The figure shows three views and two pictorial views of one solid part (mm, origin at its lowest corner). Answer the questions. Give positions to 0.01 mm unless a question says otherwise; leave off trailing zeros. Order: outer loops, then holes, each group sorted by start corner. A loop starts at its lowest first (then second) coordinate and runs counter-clockwise, first axis right, second up. Notation, with made-up numbers: (53.5, 76.25) - (97.5, 76.25) arc R23 ccw to (97.5, 86.25) - close; hole circle Ø5 at (61, 4.5). An arc over 180 degrees is marked (long way). Use a Markdown table: item, result. Add a question column.
1. A cutting plane is placed at B-B on z = 3.65. Determine the outline of the cut face in (x, y), and give its area (3 significant figures).
2. A cutting plane is placed at C-C on x = 38. Determine the outline of the cut face in (y, z).
3. A cutting plane is placed at D-D on x = 15.5. Determine the outline of the cut face in (y, z).
4. A cutting plane is placed at A-A on y = 10.5. Determine the outline of the cut face in (x, z), and give its area (3 significant figures).
5. Consider L1, parallel to X at y = 12.75, z = 2.55; L2, parallel to X at y = 10.5, z = 3.1; L3, parallel to Y at x = 38, z = 1.1. Determine where each line is inside the solid, lowest interval first.
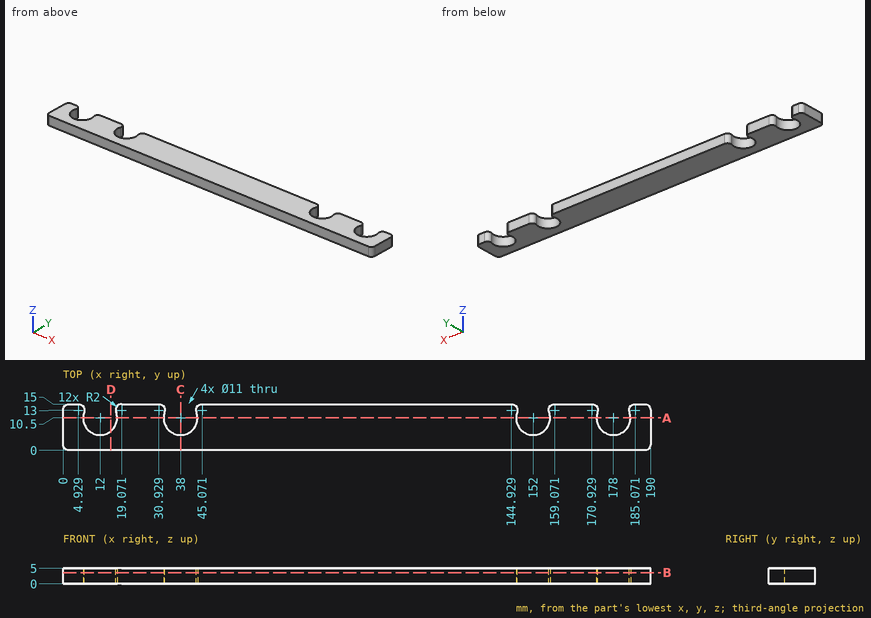
Output values:
| question | item | result |
|---|---|---|
| 1 | outline | (0, 2) arc R2 ccw to (2, 0) - (188, 0) arc R2 ccw to (190, 2) - (190, 13) arc R2 ccw to (188, 15) - (185.07, 15) arc R2 ccw to (183.19, 12.33) arc R5.5 cw (long way) to (172.81, 12.33) arc R2 ccw to (170.93, 15) - (159.07, 15) arc R2 ccw to (157.19, 12.33) arc R5.5 cw (long way) to (146.81, 12.33) arc R2 ccw to (144.93, 15) - (45.07, 15) arc R2 ccw to (43.19, 12.33) arc R5.5 cw (long way) to (32.81, 12.33) arc R2 ccw to (30.93, 15) - (19.07, 15) arc R2 ccw to (17.19, 12.33) arc R5.5 cw (long way) to (6.81, 12.33) arc R2 ccw to (4.93, 15) - (2, 15) arc R2 ccw to (0, 13) - close |
| 1 | area | 2,460 mm² |
| 2 | outline | (0, 0) - (5, 0) - (5, 5) - (0, 5) - close |
| 3 | outline | (0, 0) - (6.26, 0) - (6.26, 5) - (0, 5) - close |
| 4 | outline | (0, 0) - (6.5, 0) - (6.5, 5) - (0, 5) - close; (17.5, 0) - (32.5, 0) - (32.5, 5) - (17.5, 5) - close; (43.5, 0) - (146.5, 0) - (146.5, 5) - (43.5, 5) - close; (157.5, 0) - (172.5, 0) - (172.5, 5) - (157.5, 5) - close; (183.5, 0) - (190, 0) - (190, 5) - (183.5, 5) - close |
| 4 | area | 730 mm² |
| 5 | L1 | 0 to 6.91, 17.09 to 32.91, 43.09 to 146.91, 157.09 to 172.91, 183.09 to 190 |
| 5 | L2 | 0 to 6.5, 17.5 to 32.5, 43.5 to 146.5, 157.5 to 172.5, 183.5 to 190 |
| 5 | L3 | 0 to 5 |
